Model file for the job. Use its own axes, mm. Coordinates: 2 decimals unless noted, no trailing zeros. Loops run counter-clockwise (first coordinate to the right, second up) from the corner with the lowest first, then second, coordinate; pieces in that order, holes last. Notation, with made-up numbers: M 88.5,84.5 L 129.5,84.5 A5 cw 129.5,88.5 Z; hole C -15.5,18 d7. An arc over 180 degrees is marked long. One line per question, with ' | ' between items. Start each with the question number.
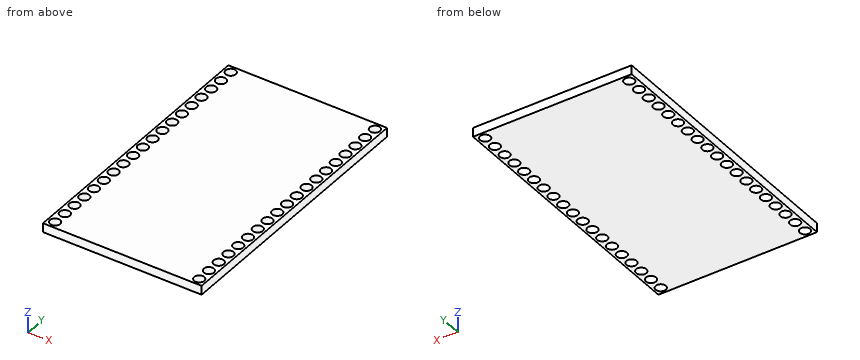
```python
from build123d import *

# Parameters (mm, degrees)
SKETCH_187_W      = 28.1
SKETCH_187_H      = 48.26
SKETCH_187_R      = 0.9
EXTRUDE_851_DEPTH = 1.6


with BuildPart() as part:
    # Sketch 187 → Extrude 851 (new body)
    with BuildSketch(Plane.XY):
        Rectangle(SKETCH_187_W, SKETCH_187_H)
        with Locations((-12.77, 22.85)):
            Circle(SKETCH_187_R, mode=Mode.SUBTRACT)
        with Locations((12.77, 22.85)):
            Circle(SKETCH_187_R, mode=Mode.SUBTRACT)
        with Locations((-12.77, 20.31)):
            Circle(SKETCH_187_R, mode=Mode.SUBTRACT)
        with Locations((12.77, 20.31)):
            Circle(SKETCH_187_R, mode=Mode.SUBTRACT)
        with Locations((-12.77, 17.77)):
            Circle(SKETCH_187_R, mode=Mode.SUBTRACT)
        with Locations((12.77, 17.77)):
            Circle(SKETCH_187_R, mode=Mode.SUBTRACT)
        with Locations((-12.77, 15.23)):
            Circle(SKETCH_187_R, mode=Mode.SUBTRACT)
        with Locations((12.77, 15.23)):
            Circle(SKETCH_187_R, mode=Mode.SUBTRACT)
        with Locations((-12.77, 12.69)):
            Circle(SKETCH_187_R, mode=Mode.SUBTRACT)
        with Locations((12.77, 12.69)):
            Circle(SKETCH_187_R, mode=Mode.SUBTRACT)
        with Locations((-12.77, 10.15)):
            Circle(SKETCH_187_R, mode=Mode.SUBTRACT)
        with Locations((12.77, 10.15)):
            Circle(SKETCH_187_R, mode=Mode.SUBTRACT)
        with Locations((-12.77, 7.61)):
            Circle(SKETCH_187_R, mode=Mode.SUBTRACT)
        with Locations((12.77, 7.61)):
            Circle(SKETCH_187_R, mode=Mode.SUBTRACT)
        with Locations((-12.77, 5.07)):
            Circle(SKETCH_187_R, mode=Mode.SUBTRACT)
        with Locations((12.77, 5.07)):
            Circle(SKETCH_187_R, mode=Mode.SUBTRACT)
        with Locations((-12.77, 2.53)):
            Circle(SKETCH_187_R, mode=Mode.SUBTRACT)
        with Locations((12.77, 2.53)):
            Circle(SKETCH_187_R, mode=Mode.SUBTRACT)
        with Locations((-12.77, -0.01)):
            Circle(SKETCH_187_R, mode=Mode.SUBTRACT)
        with Locations((12.77, -0.01)):
            Circle(SKETCH_187_R, mode=Mode.SUBTRACT)
        with Locations((-12.77, -2.55)):
            Circle(SKETCH_187_R, mode=Mode.SUBTRACT)
        with Locations((12.77, -2.55)):
            Circle(SKETCH_187_R, mode=Mode.SUBTRACT)
        with Locations((-12.77, -5.09)):
            Circle(SKETCH_187_R, mode=Mode.SUBTRACT)
        with Locations((12.77, -5.09)):
            Circle(SKETCH_187_R, mode=Mode.SUBTRACT)
        with Locations((-12.77, -7.63)):
            Circle(SKETCH_187_R, mode=Mode.SUBTRACT)
        with Locations((12.77, -7.63)):
            Circle(SKETCH_187_R, mode=Mode.SUBTRACT)
        with Locations((-12.77, -10.17)):
            Circle(SKETCH_187_R, mode=Mode.SUBTRACT)
        with Locations((12.77, -10.17)):
            Circle(SKETCH_187_R, mode=Mode.SUBTRACT)
        with Locations((-12.77, -12.71)):
            Circle(SKETCH_187_R, mode=Mode.SUBTRACT)
        with Locations((12.77, -12.71)):
            Circle(SKETCH_187_R, mode=Mode.SUBTRACT)
        with Locations((-12.77, -15.25)):
            Circle(SKETCH_187_R, mode=Mode.SUBTRACT)
        with Locations((12.77, -15.25)):
            Circle(SKETCH_187_R, mode=Mode.SUBTRACT)
        with Locations((-12.77, -17.79)):
            Circle(SKETCH_187_R, mode=Mode.SUBTRACT)
        with Locations((12.77, -17.79)):
            Circle(SKETCH_187_R, mode=Mode.SUBTRACT)
        with Locations((-12.77, -20.33)):
            Circle(SKETCH_187_R, mode=Mode.SUBTRACT)
        with Locations((12.77, -20.33)):
            Circle(SKETCH_187_R, mode=Mode.SUBTRACT)
        with Locations((-12.77, -22.87)):
            Circle(SKETCH_187_R, mode=Mode.SUBTRACT)
        with Locations((12.77, -22.87)):
            Circle(SKETCH_187_R, mode=Mode.SUBTRACT)
    extrude(amount=EXTRUDE_851_DEPTH)


solid = part.part
```
(1) Drill centre lines: line 1 (X direction, y = -8, z = 1.3); line 2 (X direction, y = -10, z = 0.95). Where is each one in solid material? Low to high. Write a range as [from, to].
(2) Band-saw the part on A-A on y = 12.69. Write the cut outline in (x, z), then the cut area to 3 significant figures.
(3) Band-saw the part on B-B on z = 0.8. Give the number of separate pieces and of enclosed holes in the cut face, then the cut area to 3 significant figures.
Computed values:
1) line 1: [-14.05, -13.59], [-11.95, 11.95], [13.59, 14.05] | line 2: [-14.05, -13.65], [-11.89, 11.89], [13.65, 14.05]
2) outline: M -14.05,0 L -13.67,0 L -13.67,1.6 L -14.05,1.6 Z; M -11.87,0 L 11.87,0 L 11.87,1.6 L -11.87,1.6 Z; M 13.67,0 L 14.05,0 L 14.05,1.6 L 13.67,1.6 Z | area: 39.2 mm^2
3) separate pieces: 1 | enclosed holes: 38 | area: 1,260 mm^2
